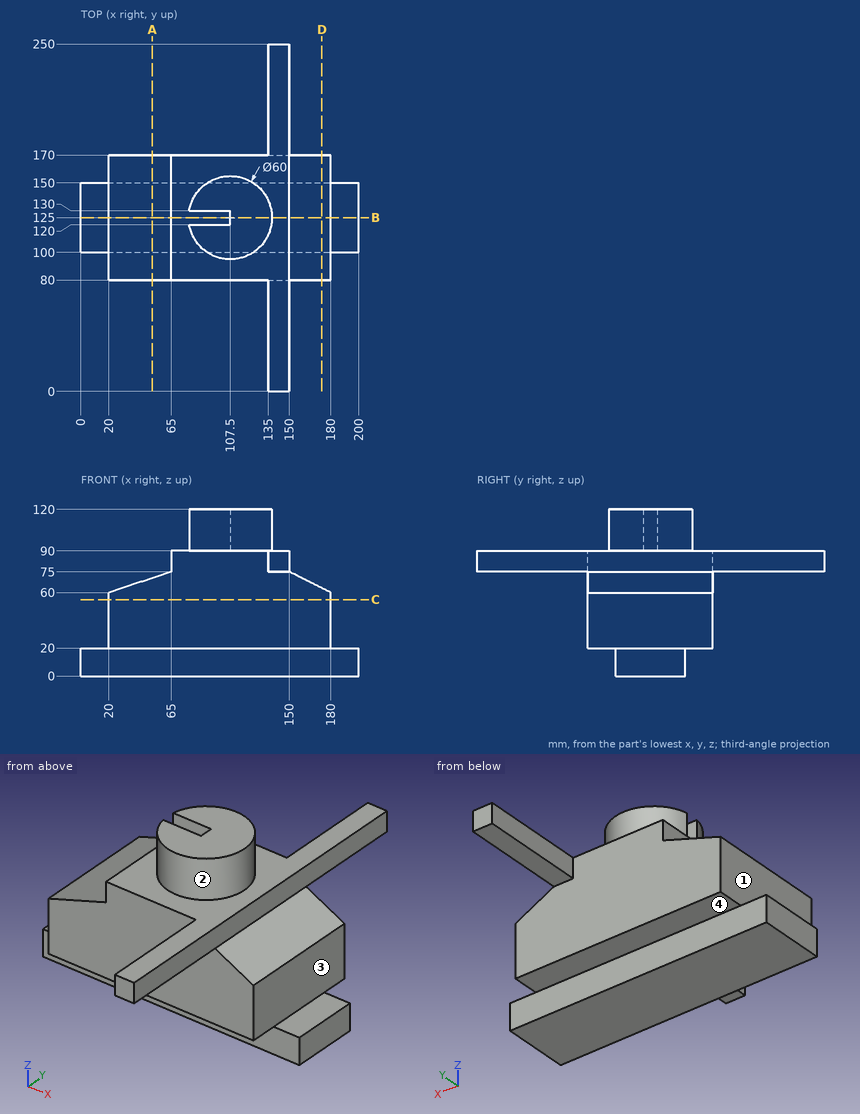
Answer from the drawing. Dimensions are ordinates in mm from the lowest x, y and z of the part. A direction names the side the tool comes from. Coordinates: 2 decimals unless noted, no trailing zeros. Write each loop counter-clockwise with the first axis right and the second up, starting at its lowest first coordinate (ties: lowest second). Pieces come first, ordered by that corner, then holes. Notation, with made-up numbers: M -39,51.25 L 11,51.25 A12 ccw 11,59.25 Z; hole C 54.5,37 d9. An arc over 180 degrees is marked long. Use a Markdown table: item, result.
Q1. Which of the six approach directions +Z, -Z, +X, -X, +Y, -Y give full straight-line access (tool end or side, diameter ignored) to the marked faces 1, 2, 3 and 4?
Answer block:
| item | result |
|---|---|
| face 1 | +Z, -X, +Y, -Y |
| face 2 | +Z |
| face 3 | +Z, +X, +Y, -Y |
| face 4 | -Z, +X, -X, +Y |
Q2. The part is cut by section C-C, the plane z = 55. Write down the section's boundary in (x, y).
Answer block:
| item | result |
|---|---|
| outline | M 20,80 L 180,80 L 180,170 L 20,170 Z |
Q3. The part is cut by section B-B, the plane y = 125. Write down the section's boundary in (x, z).
Answer block:
| item | result |
|---|---|
| outline | M 0,0 L 200,0 L 200,20 L 180,20 L 180,60 L 150,75 L 150,90 L 137.5,90 L 137.5,120 L 107.5,120 L 107.5,90 L 65,90 L 65,75 L 20,60 L 20,20 L 0,20 Z |
Q4. Each of these flat-tipped pins is pushed along its axis until it touches: pin 1 Ø1.5 at (y, z) = (108.5, 81) entering from -X; pin 2 Ø16.5 at (x, y) = (145.5, 36.5) entering from -Z; pin 3 Ø16.5 at (y, z) = (129, 80) entering from +X. Where does it stop, or does it pass through?
Answer block:
| item | result |
|---|---|
| pin 1 | stops at x = 65 |
| pin 2 | stops at z = 75 |
| pin 3 | stops at x = 156.5 |
Q5. The part is cut by section A-A, the plane x = 51.5. Write down the section's boundary in (y, z).
Answer block:
| item | result |
|---|---|
| outline | M 80,20 L 100,20 L 100,0 L 150,0 L 150,20 L 170,20 L 170,70.5 L 80,70.5 Z |
Q6. Straight lines are drawn through the part: L1, parallel to Z at x = 189, y = 144.5; L2, parallel to Y at x = 150.5, z = 52.5; L3, parallel to Y at x = 148.5, z = 19.5. For each, find the intervals that lie inside material, in ascending order. Write a range as [from, to].
Answer block:
| item | result |
|---|---|
| L1 | z = [0, 20] |
| L2 | y = [80, 170] |
| L3 | y = [100, 150] |
Q7. The part is cut by section D-D, the plane x = 173.5. Write down the section's boundary in (y, z).
Answer block:
| item | result |
|---|---|
| outline | M 80,20 L 100,20 L 100,0 L 150,0 L 150,20 L 170,20 L 170,63.25 L 80,63.25 Z |
